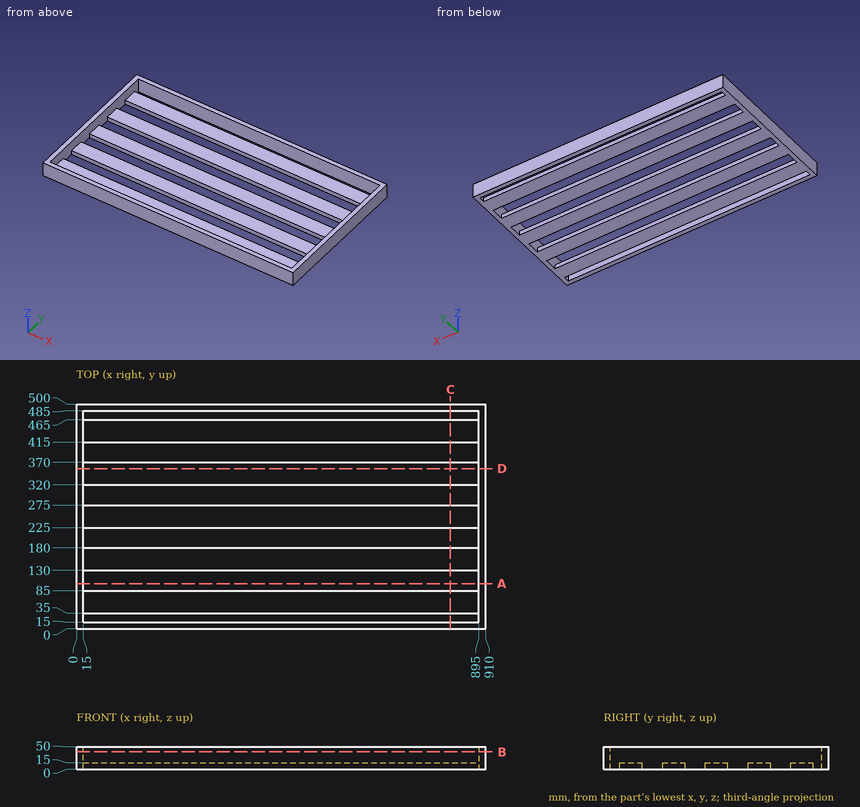
Input: dimensioned drawing with shaded views. Units: mm. Origin: part minimum x, y, z. Give positions to 0.01 mm unless a question says otherwise; leave off trailing zeros. Order: outer loops, then holes, each group sorted by start corner. A loop starts at its lowest first (then second) coordinate and runs counter-clockwise, first axis right, second up.
(1) Section query C-C (x = 831.5). Return the cut outline in (y, z), plus the area to 3 significant figures.
(2) Section query D-D (y = 356). Return the cut outline in (x, z), plus the area to 3 significant figures.
(3) Section query B-B (z = 39). Return the cut outline in (x, y), plus the area to 3 significant figures.
(4) Material intervals for line 1 along Y through (x, z) = (395.5, 30.5); line 2 along X through (y, z) = (314, 9.5); line 3 along Z through (x, y) = (81.5, 237), sorted ascending.
(5) Contact query for flat-ended pins moving along their axis: P1, Ø1, axis at x = 438.5, z = 29.5, coming from the -Y side; P2, Ø15, axis at x = 642.5, y = 248.5, coming from the +Z side. Output: stop coordinate, or through.
(6) Section query A-A (y = 100.5). Return the cut outline in (x, z).
Outcome:
1. outline: (0, 0) - (15, 0) - (15, 50) - (0, 50) - close; (35, 0) - (85, 0) - (85, 15) - (35, 15) - close; (130, 0) - (180, 0) - (180, 15) - (130, 15) - close; (225, 0) - (275, 0) - (275, 15) - (225, 15) - close; (320, 0) - (370, 0) - (370, 15) - (320, 15) - close; (415, 0) - (465, 0) - (465, 15) - (415, 15) - close; (485, 0) - (500, 0) - (500, 50) - (485, 50) - close
1. area: 5,250 mm2
2. outline: (0, 0) - (910, 0) - (910, 50) - (895, 50) - (895, 15) - (15, 15) - (15, 50) - (0, 50) - close
2. area: 14,700 mm2
3. outline: (0, 0) - (910, 0) - (910, 500) - (0, 500) - close; hole (15, 15) - (895, 15) - (895, 485) - (15, 485) - close
3. area: 41,400 mm2
4. line 1: y = 0 to 15, 485 to 500
4. line 2: x = 0 to 15, 895 to 910
4. line 3: z = 0 to 15
5. P1: stops at y = 0
5. P2: stops at z = 15
6. outline: (0, 0) - (15, 0) - (15, 50) - (0, 50) - close; (895, 0) - (910, 0) - (910, 50) - (895, 50) - close
